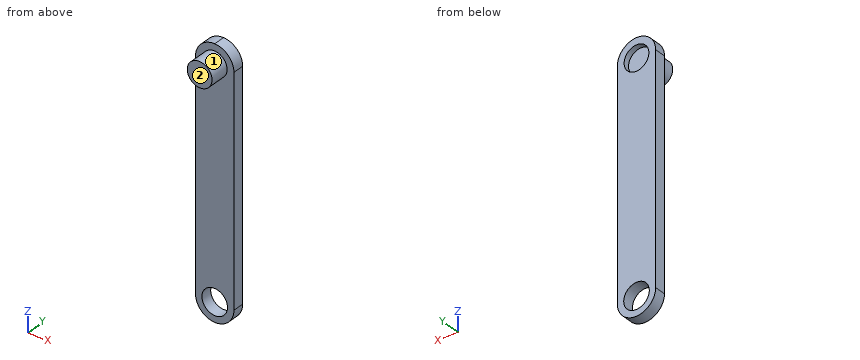
from build123d import *

# Parameters (mm, degrees)
F0_R     = 0.4064
F0_R_2   = 0.3937
F1_DEPTH = 0.1778
F2_DEPTH = 0.7874
F3_SCALE = 7.5


with BuildPart() as f1:
    # F0 (on Front) → F1 (new body, symmetric)
    with BuildSketch(Plane.XZ):
        with BuildLine():
            ThreePointArc((0, 7.7216), (-0.4310522938, 7.5430522938), (-0.6096, 7.112))
            Line((-0.6096, 7.112), (-0.6096, 0))
            ThreePointArc((-0.6096, 0), (-0.4310522938, -0.4310522938), (0, -0.6096))
            ThreePointArc((0, -0.6096), (0.4310522938, -0.4310522938), (0.6096, 0))
            Line((0.6096, 0), (0.6096, 7.112))
            ThreePointArc((0.6096, 7.112), (0.4310522938, 7.5430522938), (0, 7.7216))
        make_face()
        Circle(F0_R, mode=Mode.SUBTRACT)
        with Locations((0, 7.112)):
            Circle(F0_R_2, mode=Mode.SUBTRACT)
    extrude(amount=F1_DEPTH, both=True)

    # F0 (on Front) → F2 (join)
    with BuildSketch(Plane.XZ):
        with Locations((0, 7.112)):
            Circle(F0_R_2)
    extrude(amount=F2_DEPTH)


with BuildPart() as f1_1:
    # F3: moved
    add(f1.part.scale(F3_SCALE))


solid = f1_1.part
Build history of the part. All positions in model axes, mm. Face numbers are marked on the shaded views. A direction names the side the tool comes from. Give positions to 0.01 mm unless a question says otherwise; leave off trailing zeros. Order: outer loops, then holes, each group sorted by start corner. A loop starts at its lowest first (then second) coordinate and runs counter-clockwise, first axis right, second up. Notation, with made-up numbers: M 5,-14 L 34,-14 A12 ccw 34,6 Z; hole C 23,87.25 d1. An arc over 180 degrees is marked long. Put each result on its own line as item: value.
Item 1: 3-axis set-ups, long thin cutter, end or side, ignore diameter. For the marked faces 1 and 2: which of +Z, -Z, +X, -X, +Y, -Y reach the whole face in a straight line?
From the geometry:
face 1: -Y
face 2: +Z, -Z, +X, -X, -Y
Item 2: Flat gauge pins, fed straight in: pin 1 Ø2.5 at (x, z) = (2, 35) entering from -Y; pin 2 Ø3 at (x, z) = (0, 52.5) entering from +Y; pin 3 Ø3 at (x, y) = (-0.5, -3.5) entering from -Z. Where does each tip first touch, or does it go through?
From the geometry:
pin 1: stops at y = -1.33
pin 2: stops at y = 0
pin 3: stops at z = 50.39
Item 3: Slice it at A-A, the plane x = 1.25. Write the cut outline in (y, z), plus the area to 3 significant figures.
From the geometry:
outline: M -5.91,50.66 L -1.33,50.66 L -1.33,2.78 L 1.33,2.78 L 1.33,50.66 L 0,50.66 L 0,56.02 L 1.33,56.02 L 1.33,57.74 L -1.33,57.74 L -1.33,56.02 L -5.91,56.02 Z; M -1.33,-4.4 L 1.33,-4.4 L 1.33,-2.78 L -1.33,-2.78 Z
area: 168 mm2
Item 4: Slice it at D-D, the plane y = -2. Write the cut outline in (x, z), plus the area to 3 significant figures.
From the geometry:
outline: C 0,53.34 d5.91
area: 27.4 mm2
Item 5: Slice it at B-B, the plane y = 0.75. Write the cut outline in (x, z), plus the area to 3 significant figures.
From the geometry:
outline: M -4.57,0 A4.57 ccw 4.57,0 L 4.57,53.34 A4.57 ccw -4.57,53.34 Z; hole C 0,0 d6.1; hole C 0,53.34 d5.91
area: 497 mm2
Item 6: Probe line 1 (Z direction, x = -1.25, y = 0.25); line 2 (Y direction, x = 2, z = 31.5); line 3 (Z direction, x = 1, y = 1). List the from-to ranges inside material, lowest first. Write a range as [from, to].
From the geometry:
line 1: z = [-4.4, -2.78], [2.78, 50.66], [56.02, 57.74]
line 2: y = [-1.33, 1.33]
line 3: z = [-4.46, -2.88], [2.88, 50.56], [56.12, 57.8]
Item 7: Slice it at C-C, the plane z = 51.5. Write the cut outline in (x, y).
From the geometry:
outline: M -4.57,-1.33 L -2.31,-1.33 L -2.31,-5.91 L 2.31,-5.91 L 2.31,-1.33 L 4.57,-1.33 L 4.57,1.33 L 2.31,1.33 L 2.31,0 L -2.31,0 L -2.31,1.33 L -4.57,1.33 Z
